Autodesk Inventor part; units mm, degrees
ref_plane "YZ Plane" through (0, 0, 0) normal (1, 0, 0) x (0, 1, 0)
ref_plane "XZ Plane" through (0, 0, 0) normal (0, 1, 0) x (-1, 0, 0)
ref_plane "XY Plane" through (0, 0, 0) normal (0, 0, 1) x (1, 0, 0)
sketch "Sketch1" plane through (0, 0, 0) normal (0, 0, 1) x (1, 0, 0)
  line L0 (-6.35, -3.6662) -> (-6.35, 3.6662)
  line L1 (-6.35, 3.6662) -> (0, 7.3323)
  line L2 (0, 7.3323) -> (6.35, 3.6662)
  line L3 (6.35, 3.6662) -> (6.35, -3.6662)
  line L4 (6.35, -3.6662) -> (0, -7.3323)
  line L5 (0, -7.3323) -> (-6.35, -3.6662)
  point P0 (0, 0)
  point P1 (0, 0)
  dimension "Size" = 12.7
extrude "Extrusion1" add sketch "Sketch1" along normal mid plane 66.675
sketch "Sketch3" plane through (0, 0, 33.3375) normal (0, 0, 1) x (1, 0, 0)
  line L0 (-6.35, 3.6662) -> (0, 7.3323) construction
  line L1 (0, 7.3323) -> (6.35, 3.6662) construction
  line L2 (6.35, 3.6662) -> (6.35, -3.6662) construction
  line L3 (6.35, -3.6662) -> (0, -7.3323) construction
  line L4 (0, -7.3323) -> (-6.35, -3.6662) construction
  line L5 (-6.35, -3.6662) -> (-6.35, 3.6662) construction
  point P0 (0, 0)
hole "Hole1" at (0, 0, 33.3375) direction (0, 0, -1) diameter 5.1054 end through all
sketch "Sketch4" plane through (0, 0, 33.3375) normal (0, 0, 1) x (1, 0, 0)
  circle A0 centre (0, 0) radius 2.5527 construction
  line L0 (-6.35, 3.6662) -> (0, 7.3323) construction
  line L1 (0, 7.3323) -> (6.35, 3.6662) construction
  line L2 (6.35, 3.6662) -> (6.35, -3.6662) construction
  line L3 (6.35, -3.6662) -> (0, -7.3323) construction
  line L4 (0, -7.3323) -> (-6.35, -3.6662) construction
  line L5 (-6.35, -3.6662) -> (-6.35, 3.6662) construction
  circle A1 centre (0, 0) radius 6.8771
  circle A2 centre (0, 0) radius 8.89
  dimension "thunder" = 13.7541
  dimension "d16" = 17.78
extrude "Extrusion3" cut sketch "Sketch4" against normal through all
sketch "Sketch5" plane through (0, 0, 33.3375) normal (0, 0, 1) x (1, 0, 0)
  arc A0 (5.4616, -4.1791) -> (6.35, -2.6403) centre (0, 0) ccw
  line L0 (6.35, -2.6403) -> (6.35, 2.6403)
  arc A1 (6.35, 2.6403) -> (5.4616, 4.1791) centre (0, 0) ccw
  line L1 (5.4616, 4.1791) -> (0.8884, 6.8194)
  arc A2 (0.8884, 6.8194) -> (-0.8884, 6.8194) centre (0, 0) ccw
  line L2 (-0.8884, 6.8194) -> (-5.4616, 4.1791)
  arc A3 (-5.4616, 4.1791) -> (-6.35, 2.6403) centre (0, 0) ccw
  line L3 (-6.35, 2.6403) -> (-6.35, -2.6403)
  arc A4 (-6.35, -2.6403) -> (-5.4616, -4.1791) centre (0, 0) ccw
  line L4 (-5.4616, -4.1791) -> (-0.8884, -6.8194)
  arc A5 (-0.8884, -6.8194) -> (0.8884, -6.8194) centre (0, 0) ccw
  line L5 (0.8884, -6.8194) -> (5.4616, -4.1791)
  circle A6 centre (0, 0) radius 2.5527
  circle A7 centre (0, 0) radius 6.35
  point P0 (3.175, -5.4993)
  point P1 (-3.175, -5.4993)
  point P2 (-6.35, 0)
  point P3 (-3.175, 5.4993)
  point P4 (3.175, 5.4993)
  point P5 (6.35, 0)
  dimension "d19" = 12.7
extrude "Extrusion4" cut sketch "Sketch5" against normal blind 8.001 contours L5 A7 L0 A0 | L5 A5 L4 A7 | A7 L1 A1 L0 | L4 A4 L3 A7 | A7 L2 A2 L1 | L3 A3 L2 A7
mirror "Mirror2" about plane through (0, 0, 0) normal (0, 0, 1) of "Extrusion4"
equation "\"bearing\" = 25.4"
properties part number "GP6-009" material "Aluminum 6061"
Geometry check sheet. Reference: the model listing, model coordinates, mm. A direction names the side the tool comes from. Give positions to 0.01 mm unless a question says otherwise; leave off trailing zeros. Write each loop counter-clockwise with the first axis right and the second up, starting at its lowest first coordinate (ties: lowest second). Pieces come first, ordered by that corner, then holes. Notation, with made-up numbers: (-19, 12) - (18, 12) arc R4 ccw to (18, 17) - close; hole circle Ø11 at (10.5, 63). An arc over 180 degrees is marked (long way). Use a Markdown table: item, result.
Q1. Section check C-C, the plane z = -4. Enter the section's corners in (x, y).
Computed:
| item | result |
|---|---|
| outline | (-6.35, -2.64) arc R6.88 ccw to (-5.46, -4.18) - (-0.89, -6.82) arc R6.88 ccw to (0.89, -6.82) - (5.46, -4.18) arc R6.88 ccw to (6.35, -2.64) - (6.35, 2.64) arc R6.88 ccw to (5.46, 4.18) - (0.89, 6.82) arc R6.88 ccw to (-0.89, 6.82) - (-5.46, 4.18) arc R6.88 ccw to (-6.35, 2.64) - close; hole circle Ø5.11 at (0, 0) |
Q2. Go/stop test with flat-tipped pins: P1, Ø3, axis at x = 0, y = -2, coming from the +Z side; P2, Ø4, axis at y = 5, z = -4, coming from the +X side; P3, Ø1, axis at x = -3.5, z = 19, coming from the -Y side. Record where each tip stops, or that it passes through.
Computed:
| item | result |
|---|---|
| P1 | stops at z = 33.34 |
| P2 | stops at x = 6.19 |
| P3 | stops at y = -5.6 |
Q3. Set-up check for faces 4 (the face through (0, 6.5, -25.336)), 5 (the face through (6, 3, 25.336)), 6 (the face through (-6, 3, 25.336)): record each of +Z, -Z, +X, -X, +Y, -Y from which the full face is reachable in a straight line by a thin tool's end or side.
Computed:
| item | result |
|---|---|
| face 4 | -Z, +Y |
| face 5 | +Z, +X, +Y |
| face 6 | +Z, -X, +Y |
Q4. Thickness scan on L1, parallel to X at y = 0, z = -5.5; L2, parallel to Y at x = 0, z = -14; L3, parallel to Y at x = 2, z = -23. Record the ranges inside material, lowest first. Write a range as [from, to].
Computed:
| item | result |
|---|---|
| L1 | x = [-6.35, -2.55], [2.55, 6.35] |
| L2 | y = [-6.88, -2.55], [2.55, 6.88] |
| L3 | y = [-6.18, -1.59], [1.59, 6.18] |
Q5. Draft check along X on faces 1 (the face through (6, -3, 25.336)), 2 (the face through (-0.767, -2.435, -0.467)), 3 (the face through (6.35, 0, 0)). Enter one of: pulls with the +X half, pulls with the -X half, needs draft (parallel to the pull), parting line crosses it, or undercut.
Computed:
| item | result |
|---|---|
| face 1 | needs draft |
| face 2 | undercut |
| face 3 | pulls with the +X half |
Q6. Section check D-D, the plane x = 4.25. Enter the section's corners in (y, z).
Computed:
| item | result |
|---|---|
| outline | (-4.88, -25.34) - (-4.72, -25.34) - (-4.72, -33.34) - (4.72, -33.34) - (4.72, -25.34) - (4.88, -25.34) - (4.88, 25.34) - (4.72, 25.34) - (4.72, 33.34) - (-4.72, 33.34) - (-4.72, 25.34) - (-4.88, 25.34) - close |
Q7. Section check B-B, the plane y = 1.5. Enter the section's corners in (x, z).
Computed:
| item | result |
|---|---|
| outline | (-6.35, -25.34) - (-6.17, -25.34) - (-6.17, -33.34) - (-2.07, -33.34) - (-2.07, 33.34) - (-6.17, 33.34) - (-6.17, 25.34) - (-6.35, 25.34) - close; (2.07, -33.34) - (6.17, -33.34) - (6.17, -25.34) - (6.35, -25.34) - (6.35, 25.34) - (6.17, 25.34) - (6.17, 33.34) - (2.07, 33.34) - close |
Q8. Section check A-A, the plane x = 0. Enter the section's corners in (y, z), then the cut area to 3 significant figures.
Computed:
| item | result |
|---|---|
| outline | (-6.88, -25.34) - (-6.35, -25.34) - (-6.35, -33.34) - (-2.55, -33.34) - (-2.55, 33.34) - (-6.35, 33.34) - (-6.35, 25.34) - (-6.88, 25.34) - close; (2.55, -33.34) - (6.35, -33.34) - (6.35, -25.34) - (6.88, -25.34) - (6.88, 25.34) - (6.35, 25.34) - (6.35, 33.34) - (2.55, 33.34) - close |
| area | 560 mm² |
